```python
from build123d import *

# Parameters (mm, degrees)
SKETCH1_R        = 2.4585
BASENUT_DEPTH    = 5
ENDCHAMFER2_SIZE = 0.166666667


with BuildPart() as part:
    # Sketch1 → BaseNut (new body)
    with BuildSketch(Plane.XY):
        Polygon((2.886751346, -5), (5.773502692, 0), (2.886751346, 5), (-2.886751346, 5), (-5.773502692, 0), (-2.886751346, -5), align=None)
        Circle(SKETCH1_R, mode=Mode.SUBTRACT)
    extrude(amount=-BASENUT_DEPTH)

    # Sketch2 → Chamfer1 (revolve, cut)
    with BuildSketch(Plane(origin=(15.04811501, 0, -16.706149795), x_dir=(0, 0, -1), z_dir=(0, 1, 0))):
        Polygon((-12.152731783, 20.821617702), (-11.706149795, 20.04811501), (-11.706149795, 20.821617702), align=None)
    revolve(axis=Axis((0, 0, 7.016501752), (0, 0, -1)), mode=Mode.SUBTRACT)

    # Sketch6 → EndChamfer1 (revolve, cut)
    with BuildSketch(Plane(origin=(-9.197458863, 0, -10.252541137), x_dir=(0, 0, 1), z_dir=(0, 1, 0))):
        Polygon((5.252541137, 11.655958863), (5.252541137, 12.572458863), (5.781682659, 11.655958863), align=None)
    revolve(axis=Axis((0, 0, 13.104863586), (0, 0, -1)), mode=Mode.SUBTRACT)

    # Sketch5 → Chamfer2 (revolve, cut)
    with BuildSketch(Plane(origin=(-14.793032735, 0, -16.96123207), x_dir=(0, 0, 1), z_dir=(0, 1, 0)), mode=Mode.PRIVATE) as chamfer2_sk:
        Polygon((16.96123207, 19.243032735), (16.96123207, 20.566535427), (16.197107435, 20.566535427), align=None)
    revolve(chamfer2_sk.sketch.rotate(Axis((0, 0, -39.536013381), (0, 0, 1)), 180), axis=Axis((0, 0, -39.536013381), (0, 0, 1)), mode=Mode.SUBTRACT)

    # EndChamfer2
    endchamfer2_edges = [part.edges().sort_by_distance(p)[0] for p in [
        (-2.4585, 0, 0),
    ]]
    chamfer(endchamfer2_edges, length=ENDCHAMFER2_SIZE)


solid = part.part
```
The listing builds one solid part. Answer for the finished solid, in the listing's coordinates (mm). Coordinates: 2 decimals unless noted, no trailing zeros. Loops run counter-clockwise (first coordinate to the right, second up) from the corner with the lowest first, then second, coordinate; pieces in that order, holes last. Notation, with made-up numbers: M -12,13 L -6,13 A6 ccw -6,17 Z; hole C 51,84 d2. An arc over 180 degrees is marked long. Answer as CSV lines item,"result". Start each with the question number.
(1) The part is cut by section A-A (z = -1.25). Give the vertices of the cut face in (x, y).
(2) Given pin 1 (1 mm diameter, centred on y = 3.5, z = -2.5, fed in from +X), flat-ended and moving along its own axis, determine where the tip first touches the part or whether it passes through.
(3) The mould has two halves that part along Y. Classify faces 1 (the conical face through (-2.58, -4.5, -4.89)), 2 (the cylindrical face through (2.345, 0.738, -2.289)), 3 (the conical face through (2.58, 4.5, -4.89)), 4 (the conical face through (5.184, 0.013, -4.894)): pulls with the +Y half, pulls with the -Y half, needs draft (parallel to the pull), parting line crosses it, or undercut.
(4) Find the intervals of material crossed by L1, parallel to Y at x = 0, z = -2.9; L2, parallel to Z at x = 5, y = 0; L3, parallel to Y at x = 1.75, z = -0.55, in increasing order. Write a range as [from, to].
Determined:
1,outline,"M -5.77,0 L -2.89,-5 L 2.89,-5 L 5.77,0 L 2.89,5 L -2.89,5 Z; hole C 0,0 d4.92"
2,pin 1,"x = 4.04"
3,face 1,"pulls with the -Y half"
3,face 2,"undercut"
3,face 3,"pulls with the +Y half"
3,face 4,"parting line crosses it"
4,L1,"[-5, -2.46], [2.46, 5]"
4,L2,"[-5, -0.32]"
4,L3,"[-5, -1.73], [1.73, 5]"
